Check sheet for the modelled part. Datum: model origin and axes. Units: mm. A direction names the side the tool comes from. Give positions to 0.01 mm unless a question says otherwise; leave off trailing zeros. Write each loop counter-clockwise with the first axis right and the second up, starting at its lowest first coordinate (ties: lowest second). Pieces come first, ordered by that corner, then holes.
from build123d import *
from build123d.topology import SkipClean

# Parameters (mm, degrees)
EXTRUDE_THIN1_DEPTH = 10
FILLET1_R           = 4
CUT_EXTRUDE1_START  = -1.8
CUT_EXTRUDE1_DEPTH  = 44.155533586
CUT_EXTRUDE7_START  = -10
SKETCH10_R          = 3.75
CUT_EXTRUDE7_DEPTH  = 10
SKETCH4_R           = 1
CUT_EXTRUDE2_DEPTH  = 6
FILLET2_R           = 4
CUT_EXTRUDE5_START  = -1.8
CUT_EXTRUDE5_DEPTH  = 32.937960909
CUT_EXTRUDE9_START  = -10
SKETCH12_R          = 3.75
CUT_EXTRUDE9_DEPTH  = 10


with BuildPart() as part:
    # Sketch1 → Extrude-Thin1 (new body)
    with BuildSketch(Plane.XY):
        Polygon((-17.5, -20), (-17.5, 0), (17.5, 0), (17.5, -20), (21.5, -20), (21.5, 4), (-21.5, 4), (-21.5, -20), align=None)
    extrude(amount=EXTRUDE_THIN1_DEPTH)

    # Fillet1
    fillet1_edges = [part.edges().sort_by_distance(p)[0] for p in [
        (-21.5, 4, 5),
        (21.5, 4, 5),
        (17.5, 0, 5),
        (-17.5, 0, 5),
    ]]
    fillet(fillet1_edges, radius=FILLET1_R)

    # Sketch3 → Cut-Extrude1 (cut, through all)
    with BuildSketch(Plane.ZY.offset(-17.5).offset(CUT_EXTRUDE1_START)):
        with BuildLine():
            Line((1.324257426, -15.307425743), (1.25, -16.05))
            ThreePointArc((1.25, -16.05), (5, -19.8), (8.75, -16.05))
            Line((8.75, -16.05), (8.675742574, -15.307425743))
            Line((8.675742574, -15.307425743), (7.545, -4))
            Line((7.545, -4), (2.455, -4))
            Line((2.455, -4), (1.324257426, -15.307425743))
        make_face()
        with BuildLine():
            Line((2.9, 0.45), (2.455, -4))
            Line((2.455, -4), (7.545, -4))
            Line((7.545, -4), (7.1, 0.45))
            ThreePointArc((7.1, 0.45), (5, 2.55), (2.9, 0.45))
        make_face()
    extrude(amount=-CUT_EXTRUDE1_DEPTH, mode=Mode.SUBTRACT)

    # Sketch10 → Cut-Extrude7 (cut)
    with BuildSketch(Plane(origin=(19.3, 0, 0), x_dir=(0, 0, -1), z_dir=(1, 0, 0)).offset(CUT_EXTRUDE7_START)):
        with Locations(Location((-5, -16.05, 0), (0, 0, 270))):
            Circle(SKETCH10_R)
    extrude(amount=CUT_EXTRUDE7_DEPTH, mode=Mode.SUBTRACT)

    # Sketch4 → Cut-Extrude2 (cut)
    with BuildSketch(Plane.ZY.offset(21.5)):
        with Locations(Location((5, -16.05, 0), (0, 0, 270))):
            Circle(SKETCH4_R)
    extrude(amount=-CUT_EXTRUDE2_DEPTH, mode=Mode.SUBTRACT)

    # Fillet2
    fillet2_edges = [part.edges().sort_by_distance(p)[0] for p in [
        (-19.5, -20, 10),
        (-19.5, -20, 0),
    ]]
    fillet(fillet2_edges, radius=FILLET2_R)

    # Sketch8 → Cut-Extrude5 (cut, through all)
    with BuildSketch(Plane(origin=(0, 4, 0), x_dir=(1, 0, 0), z_dir=(0, 1, 0)).offset(CUT_EXTRUDE5_START)):
        with BuildLine():
            Line((1.034235097, -8.604560689), (16, -6.5))
            ThreePointArc((16, -6.5), (17.5, -5), (16, -3.5))
            Line((16, -3.5), (1.034235097, -1.395439311))
            ThreePointArc((1.034235097, -1.395439311), (-3.75, -5), (1.034235097, -8.604560689))
        make_face()
    extrude(amount=-CUT_EXTRUDE5_DEPTH, mode=Mode.SUBTRACT)

    # Sketch12 → Cut-Extrude9 (cut)
    with SkipClean():  # the faces are left unmerged after this step: merging them gives an invalid solid
        with BuildSketch(Plane.XZ.offset(-2.2).offset(CUT_EXTRUDE9_START)):
            with Locations(Location((0, 5, 0), (0, 0, 73.990542285))):
                Circle(SKETCH12_R)
        extrude(amount=CUT_EXTRUDE9_DEPTH, mode=Mode.SUBTRACT)


solid = part.part
1) Scan lines: L1, parallel to X at y = -7.5, z = 7; L2, parallel to Z at x = 0, y = 1.35; L3, parallel to X at y = -8.75, z = 9.25. Record each from-to range of solid material in increasing order.
2) Sectioned sample at B-B on x = 0. Record the boundary of the cut face in (y, z), then the cut area to 3 significant figures.
3) Draft check along X on faces 1 (the cylindrical face through (16.297, -1.141, 1.979)), 2 (the cylindrical face through (-20.297, 2.859, 5.07)), 3 (the flat face through (19.3, -6, 5)), 4 (the flat face through (19, -20, 5)). Enter one of: +X half, -X half, draft (parallel to the pull), parting line (faces both ways), or undercut.
4) Sectioned sample at A-A on y = -6.75. Record the boundary of the cut face in (x, z), then the cut area to 3 significant figures.
5) Sectioned sample at D-D on x = 5. Record the boundary of the cut face in (y, z), then the cut area to 3 significant figures.
6) Gauge pin test, flat ends, axial feed: pin 1 (1.5 mm diameter, centred on x = 6.5, z = 4.5, fed in from -Y); pin 2 (4.5 mm diameter, centred on y = -16.05, z = 5, fed in from -X); pin 3 (3 mm diameter, centred on x = -6.5, z = 6, fed in from -Y); pin 4 (3 mm diameter, centred on y = -14, z = 3.5, fed in from +X). Record the tip position at first contact, or that the pin passes through.
7) Access from +Z, -Z, +X, -X, +Y, -Y to the whole of each face (thin tool, end or side, straight path). Record for faces 5 (the flat face through (-17.5, -12, 5)), 6 (the cylindrical face through (17.5, -0.2, 5)), 7 (the cylindrical face through (-19.472, -18.859, 8.797)), 8 (the cylindrical face through (-19.472, -18.797, 1.141)), 9 (the cylindrical face through (19.03, -19.53, 3.6)).
8) Sectioned sample at C-C on y = -10.75. Record the boundary of the cut face in (x, z), then the cut area to 3 significant figures.
Answers below:
1. L1: x = -21.5 to -17.5, 17.5 to 19.3
1. L2: z = 0 to 1.25, 8.75 to 10
1. L3: x = -21.5 to -17.5, 17.5 to 21.5
2. outline: (0, 0) - (4, 0) - (4, 1.25) - (0, 1.25) - close; (0, 8.75) - (4, 8.75) - (4, 10) - (0, 10) - close
2. area: 10.0 mm2
3. face 1: undercut
3. face 2: -X half
3. face 3: +X half
3. face 4: draft
4. outline: (-21.5, 0) - (-17.5, 0) - (-17.5, 10) - (-21.5, 10) - close; (17.5, 0) - (21.5, 0) - (21.5, 2.18) - (19.3, 2.18) - (19.3, 7.82) - (21.5, 7.82) - (21.5, 10) - (17.5, 10) - close
4. area: 67.6 mm2
5. outline: (0, 0) - (4, 0) - (4, 10) - (0, 10) - (0, 8.05) - (2.2, 8.05) - (2.2, 1.95) - (0, 1.95) - close
5. area: 26.6 mm2
6. pin 1: stops at y = 2.2
6. pin 2: stops at x = -21.5
6. pin 3: stops at y = 0
6. pin 4: stops at x = 19.3
7. face 5: +Z, -Z, -Y
7. face 6: -Y
7. face 7: +Z, -X, -Y
7. face 8: -Z, -X, -Y
7. face 9: +X
8. outline: (-21.5, 0) - (-17.5, 0) - (-17.5, 10) - (-21.5, 10) - close; (17.5, 0) - (21.5, 0) - (21.5, 1.78) - (19.3, 1.78) - (19.3, 8.22) - (21.5, 8.22) - (21.5, 10) - (17.5, 10) - close
8. area: 65.8 mm2
